Check sheet for the modelled part. Datum: model origin and axes. Units: mm. Coordinates: 2 decimals unless noted, no trailing zeros. Loops run counter-clockwise (first coordinate to the right, second up) from the corner with the lowest first, then second, coordinate; pieces in that order, holes last.
from build123d import *

# Parameters (mm, degrees)
EXTRUDE_1_DEPTH     = 520
SKETCH_2_R          = 2
CUT_EXTRUDE_1_DEPTH = 38.499979182


with BuildPart() as part:
    # 草圖1 → 填料-伸長1 (new body)
    with BuildSketch(Plane.XY):
        Polygon((0, 0), (17.69379362, -17.661530719), (0.032262901, -35.355324339), (-17.661530719, -17.69379362), align=None)
        Polygon((0.001935774, -2.12131946), (-15.540211259, -17.691857846), (0.030327127, -33.234004879), (15.57247416, -17.663466493), align=None, mode=Mode.SUBTRACT)
    extrude(amount=EXTRUDE_1_DEPTH)

    # 草圖2 → 除料-伸長1 (cut, through all)
    with BuildSketch(Plane(origin=(0, 0, 0), x_dir=(0.707751745, -0.706461229, 0), z_dir=(0.706461229, 0.707751745, 0))):
        with Locations((12.5, -455)):
            Circle(SKETCH_2_R)
        with Locations((12.5, -495)):
            Circle(SKETCH_2_R)
        with Locations((12.5, -25)):
            Circle(SKETCH_2_R)
        with Locations((12.5, -65)):
            Circle(SKETCH_2_R)
    extrude(amount=-CUT_EXTRUDE_1_DEPTH, mode=Mode.SUBTRACT)


solid = part.part
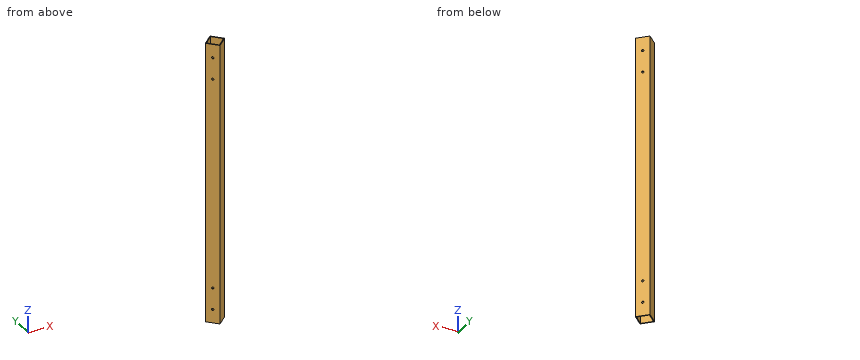
(1) Section check A-A, the plane z = 125. Enter the section's corners in (x, y).
(2) Gauge pin test, flat ends, axial feed: P1, Ø5, axis at y = -15, z = 410, coming from the -X side; P2, Ø1, axis at y = -15, z = 72, coming from the +X side; P3, Ø3, axis at x = 12.5, z = 273.5, coming from the -Y side. Record the tip position at first contact, or that the pin passes through.
(3) Scan lines: line 1 along Y through (x, z) = (-4, 290.5); line 2 along X through (y, z) = (-6, 253.5); line 3 along X through (y, z) = (-15.5, 313). Record each from-to range of solid material in increasing order.
Determined:
1. outline: (-17.66, -17.69) - (0.03, -35.36) - (17.69, -17.66) - (0, 0) - close; hole (-15.54, -17.69) - (0.03, -33.23) - (15.57, -17.66) - (0, -2.12) - close
2. P1: stops at x = -17.47
2. P2: stops at x = 15.53
2. P3: stops at y = -24.37
3. line 1: y = -31.33 to -29.21, -6.13 to -4.01
3. line 2: x = -5.99 to -3.87, 3.89 to 6.01
3. line 3: x = -15.47 to -13.35, 13.41 to 15.53
